```python
from build123d import *

# Parameters (mm, degrees)
SKIZZE2_W = 0.5
SKIZZE2_H = 0.2


with BuildPart() as part:
    # Skizze1 → Rotation1 (revolve)
    with BuildSketch(Plane.XY):
        Polygon((0, 0), (0, 19), (78, 19), (78, 6), (80, 6), (80, 0), align=None)
    revolve(axis=Axis((0, 0, 0), (1, 0, 0)))

    # Skizze2 → Schnitt-Rotation1 (revolve, cut)
    with BuildSketch(Plane.XY):
        with Locations((74.75, 18.9)):
            Rectangle(SKIZZE2_W, SKIZZE2_H)
    revolve(axis=Axis((0, 0, 0), (1, 0, 0)), mode=Mode.SUBTRACT)


solid = part.part
```
Here's how the part is built. I have some questions about the finished solid (model axes, mm). A direction names the side the tool comes from. Give positions to 0.01 mm unless a question says otherwise; leave off trailing zeros. Loops run counter-clockwise (first coordinate to the right, second up) from the corner with the lowest first, then second, coordinate; pieces in that order, holes last. Notation, with made-up numbers: M 76,-35.5 L 120,-35.5 A17 ccw 120,-18.5 Z; hole C -26.75,65 d5. An arc over 180 degrees is marked long. Put each result on its own line as item: value. Start each with the question number.
(1) I need wall thicknesses on line 1 along X through (y, z) = (12.5, -11); line 2 along Z through (x, y) = (12, 4); line 3 along Z through (x, y) = (68, -12). Which ranges of each line are inside material? Lowest first, please. Write a range as [from, to].
(2) If we mould it in two halves opening along X, with no side actions, what happens to faces 1 (the cylindrical face through (74.754, 8.675, -16.679)), 2 (the flat face through (0, 0, 0)), 3 (the cylindrical face through (37.772, 8.767, -16.856)), 4 (the flat face through (78, -4.5, 4.5))? For each: +X half, -X half, draft (parallel to the pull), parting line (faces both ways), or undercut.
(3) I want a section at D-D on z = -12. Please give me the cut outline in (x, y).
(4) Will these pins go through, and if not, where does the flat tip stop? pin 1 Ø1.5 at (x, z) = (10, 10) entering from +Y; pin 2 Ø5 at (x, z) = (68, -14) entering from +Y; pin 3 Ø1.5 at (x, y) = (10, 3) entering from -Z.
(5) For faces 5 (the cylindrical face through (79, -6, 0)), 6 (the cylindrical face through (76.521, 8.767, -16.856)), which set-ups out of +Z, -Z, +X, -X, +Y, -Y let a thin tool reach every point of the face, with its end or its side?
(6) I want a section at C-C on x = 55. Please give me the cut outline in (y, z).
(7) I want a section at A-A on y = 0. Please give me the cut outline in (x, z), then the cut area to 3 significant figures.
Answer block:
1. line 1: [0, 78]
1. line 2: [-18.57, 18.57]
1. line 3: [-14.73, 14.73]
2. face 1: undercut
2. face 2: -X half
2. face 3: draft
2. face 4: +X half
3. outline: M 0,-14.73 L 74.5,-14.73 L 74.5,-14.47 L 75,-14.47 L 75,-14.73 L 78,-14.73 L 78,14.73 L 75,14.73 L 75,14.47 L 74.5,14.47 L 74.5,14.73 L 0,14.73 Z
4. pin 1: y = 16.6
4. pin 2: y = 15.12
4. pin 3: z = -18.87
5. face 5: +X
5. face 6: +X, -X
6. outline: C 0,0 d38
7. outline: M 0,-19 L 74.5,-19 L 74.5,-18.8 L 75,-18.8 L 75,-19 L 78,-19 L 78,-6 L 80,-6 L 80,6 L 78,6 L 78,19 L 75,19 L 75,18.8 L 74.5,18.8 L 74.5,19 L 0,19 Z
7. area: 2,990 mm^2
